Autodesk Inventor part; units mm, degrees
ref_plane "YZ Plane" through (0, 0, 0) normal (1, 0, 0) x (0, 1, 0)
ref_plane "XZ Plane" through (0, 0, 0) normal (0, 1, 0) x (-1, 0, 0)
ref_plane "XY Plane" through (0, 0, 0) normal (0, 0, 1) x (1, 0, 0)
sketch "草图1" plane through (0, 0, 0) normal (1, 0, 0) x (0, 1, 0)
  circle A0 centre (0, 0) radius 40
  dimension "d0" = 80
extrude "拉伸1" add sketch "草图1" along normal blind 40
sketch "草图2" plane through (40, 0, 0) normal (1, 0, 0) x (0, 0, -1)
  circle A0 centre (0, 0) radius 3
  dimension "d3" = 6
extrude "拉伸2" cut sketch "草图2" against normal through all
fillet "圆角1" radius 2 1 edges at (0, -40, 0)
fillet "圆角2" radius 2 1 edges at (40, -40, 0)
properties part number "轮子"
For this review, take the finished solid that the model builds, in its own axes (mm). Round coordinates to 2 decimals unless told otherwise and drop trailing zeros. Loops run counter-clockwise (first coordinate to the right, second up) from the corner with the lowest first, then second, coordinate; pieces in that order, holes last. Notation, with made-up numbers: (60, 16.25) - (87, 16.25) arc R22 ccw to (87, 22.25) - close; hole circle Ø10 at (-37.75, 39). An arc over 180 degrees is marked (long way). Put each result on its own line as item: value. Start each with the question number.
1. Consider section C-C on x = 32.5. State the section outline as (y, z) points.
2. Consider section A-A on y = 0. State the section outline as (x, z) points.
3. For probe 1 along Y at (x, z) = (5.5, -1); probe 2 along Z at (x, y) = (31.5, 2); probe 3 along Z at (x, y) = (12.5, 23), list the stretches that pass through material, from the lowest coordinate up. Write a range as [from, to].
4. Mouldability with a two-part tool opening along Y and no side actions: class faces 1 (the flat face through (0, -1, -8)), 2 (the cylindrical face through (20, 0, 3)), 3 (the cylindrical face through (19.75, -8.67, 39.05)) as +Y half, -Y half, draft (parallel to the pull), parting line (faces both ways), or undercut.
5. Insertion check: P1, Ø3, axis at x = 18, z = -14.5, coming from the +Y side; P2, Ø5.5, axis at y = 0, z = 0, coming from the -X side; P3, Ø3, axis at x = 26, z = -3.5, coming from the +Y side; P4, Ø10, axis at x = 17, z = -14, coming from the -Y side. Each pin has a flat end and moves straight along its axis. Give the tip position at first contact, or say it passes through.
Result sheet:
1. outline: circle Ø80 at (0, 0); hole circle Ø6 at (0, 0)
2. outline: (0, -38) arc R2 ccw to (2, -40) - (38, -40) arc R2 ccw to (40, -38) - (40, -3) - (0, -3) - close; (0, 3) - (40, 3) - (40, 38) arc R2 ccw to (38, 40) - (2, 40) arc R2 ccw to (0, 38) - close
3. probe 1: [-39.99, -2.83], [2.83, 39.99]
3. probe 2: [-39.95, -2.24], [2.24, 39.95]
3. probe 3: [-32.73, 32.73]
4. face 1: draft
4. face 2: undercut
4. face 3: parting line
5. P1: y = 37.83
5. P2: through
5. P3: y = 39.95
5. P4: y = -38.97
